from build123d import *

# Parameters (mm, degrees)
EXTRUDE_1_DEPTH     = 3
CUT_EXTRUDE_3_DEPTH = 5
FILLET_5_R          = 3


with BuildPart() as part:
    # Эскиз2 → Бобышка-Вытянуть1 (new body)
    with BuildSketch(Plane(origin=(0, 0, 0), x_dir=(1, 0, 0), z_dir=(0, 1, 0))):
        with BuildLine():
            Line((97.975465344, 20.020194571), (106.165355323, 28.790924422))
            ThreePointArc((106.165355323, 28.790924422), (28.149005714, 106.337356923), (-78.01634961, 77.546432501))
            Line((-78.01634961, 77.546432501), (-66.325729759, 74.83914465))
            ThreePointArc((-66.325729759, 74.83914465), (31.649735585, 94.859339221), (97.975465344, 20.020194571))
        make_face()
    extrude(amount=EXTRUDE_1_DEPTH)

    # Эскиз3 → Вырез-Вытянуть3 (cut)
    with BuildSketch(Plane(origin=(0, 3, 0), x_dir=(1, 0, 0), z_dir=(0, 1, 0))):
        Polygon((36.108993933, 94.920117092), (43.969168032, 92.583952898), (45.450638009, 97.568453546), (37.59046391, 99.90461774), align=None)
        Polygon((13.736254487, 101.569638102), (21.596428586, 99.233473909), (23.077898562, 104.217974556), (15.217724464, 106.55413875), align=None)
    extrude(amount=-CUT_EXTRUDE_3_DEPTH, mode=Mode.SUBTRACT)

    # Скругление5
    fillet_5_edges = [part.edges().sort_by_distance(p)[0] for p in [
        (-66.325729759, 1.5, -74.83914465),
        (-78.01634961, 1.5, -77.546432501),
        (106.165355323, 1.5, -28.790924422),
        (97.975465344, 1.5, -20.020194571),
    ]]
    fillet(fillet_5_edges, radius=FILLET_5_R)


solid = part.part
CAD build for the part. Positions are in the model's coordinates, mm. Round coordinates to 2 decimals unless told otherwise and drop trailing zeros. Loops run counter-clockwise (first coordinate to the right, second up) from the corner with the lowest first, then second, coordinate; pieces in that order, holes last.
(1) Cut at C-C (x = 47.5). Give the cut face in (y, z), plus the area to 3 significant figures.
(2) Cut at D-D (z = -79). Give the cut face in (x, y), plus the area to 3 significant figures.
(3) Cut at B-B (z = -88.5). Give the cut face in (x, y).
(4) Wall check: line 1 along X through (y, z) = (1.35, -91.5); line 2 along X through (y, z) = (1.85, -83.5) (3 decimals); line 3 along Z through (x, y) = (-0.5, 2.55). Give the ranges that are in metal, low to high.
(5) Cut at A-A (y = 2.5). Give the cut face in (x, z).
(6) Two-plate mould, pull along X, no slides. Class faces 1 (the flat face through (103.39, 1.48, -25.82)), 2 (the cylindrical face through (31.54, 1.48, -105.38)), 3 (the cylindrical face through (28, 1, -96)), 4 (the flat face through (22, 0, -99)): +X half, -X half, draft (parallel to the pull), parting line (faces both ways), or undercut.
Findings below:
1. outline: (0, -99.22) - (3, -99.22) - (3, -88) - (0, -88) - close
1. area: 33.7 mm2
2. outline: (-74.92, 0) - (-61.31, 0) - (-61.31, 3) - (-74.92, 3) - close; (61.31, 0) - (76.54, 0) - (76.54, 3) - (61.31, 3) - close
2. area: 86.5 mm2
3. outline: (-65.33, 0) - (-46.56, 0) - (-46.56, 3) - (-65.33, 3) - close; (46.56, 0) - (65.33, 0) - (65.33, 3) - (46.56, 3) - close
4. line 1: x = -61.06 to -40.35, 40.35 to 61.06
4. line 2: x = -71.608 to -55.025, 55.025 to 71.608
4. line 3: z = -110 to -100
5. outline: (-73.95, -81.44) arc R110 ccw to (105.71, -30.44) arc R3 ccw to (105.02, -27.56) - (101.81, -24.13) arc R3 ccw to (96.72, -25.41) arc R100 cw to (-65.19, -75.83) arc R3 ccw to (-67.82, -75.19) - (-72.61, -76.29) arc R3 ccw to start; hole (13.74, -101.57) - (15.22, -106.55) - (23.08, -104.22) - (21.6, -99.23) - close; hole (36.11, -94.92) - (37.59, -99.9) - (45.45, -97.57) - (43.97, -92.58) - close
6. face 1: +X half
6. face 2: parting line
6. face 3: undercut
6. face 4: draft
